For this review, use the dimensioned drawing (mm, ordinates from the lowest corner) and the shaded views. A direction names the side the tool comes from. Coordinates: 2 decimals unless noted, no trailing zeros. Loops run counter-clockwise (first coordinate to the right, second up) from the corner with the lowest first, then second, coordinate; pieces in that order, holes last. Notation, with made-up numbers: M -36,24.5 L -5,24.5 A31 ccw -5,49.5 Z; hole C 84,60 d5. An arc over 180 degrees is marked long. Write each question's results on one line, items separated by ' | '. Start each with the question number.
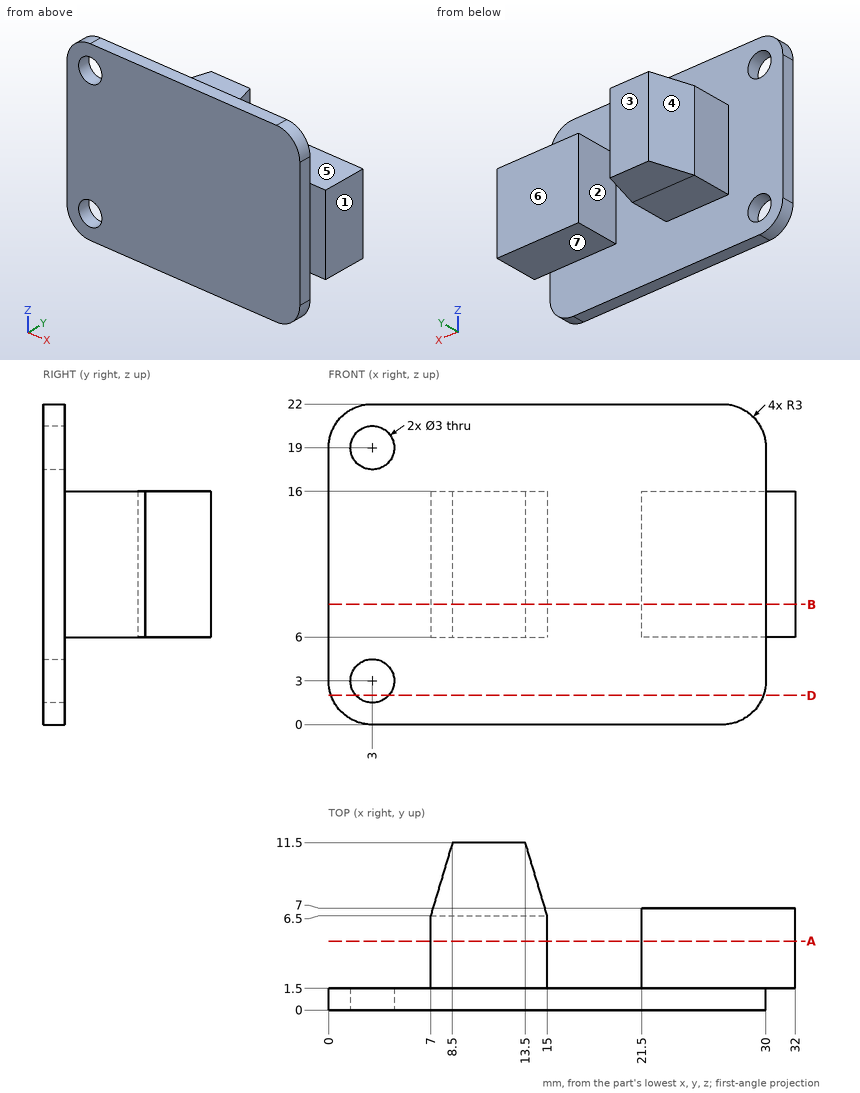
Q1. For the marked faces 5, 6 and 7, list the 3-axis set-ups (+Z, -Z, +X, -X, +Y, -Y) from which the entire face can be reached by the end or side of a thin tool; tool diameter is ignored.
Q2. The part is to be moulded in two halves that separate along X. For the marked faces 1, 2, 3 and 4, say which applies: pulls with the +X half, pulls with the -X half, needs draft (parallel to the pull), parting line crosses it, or undercut.
Q3. Take a section at B-B, the plane z = 8.25. Give the boundary of the cut face in (x, y).
Q4. Insertion check: P1, Ø8, axis at x = 27.5, z = 11, coming from the +Y side; P2, Ø0.6, axis at x = 31, z = 13, coming from the -Y side; P3, Ø2.5, axis at y = 4.5, z = 9.5, coming from the -X side. Each pin has a flat end and moves straight along its axis. Give the tip position at first contact, or say it passes through.
Q5. Take a section at D-D, the plane z = 2. Give the boundary of the cut face in (x, y), then the cut area to 3 significant figures.
Q6. Take a section at A-A, the plane y = 4.75. Give the boundary of the cut face in (x, z).
Q7. To check wall thickness, follow line 1 along X through (y, z) = (3, 11.75); line 2 along X through (y, z) = (0.6, 19); line 3 along Y through (x, z) = (7, 4). State the ranges of each line that lie inside material, in increasing order.
Results:
1) face 5: +Z, +X, -X, +Y | face 6: +Z, -Z, +X, +Y | face 7: -Z, +X, -X, +Y
2) face 1: pulls with the +X half | face 2: undercut | face 3: needs draft | face 4: pulls with the -X half
3) outline: M 0,0 L 30,0 L 30,1.5 L 32,1.5 L 32,7 L 21.5,7 L 21.5,1.5 L 15,1.5 L 15,6.5 L 13.5,11.5 L 8.5,11.5 L 7,6.5 L 7,1.5 L 0,1.5 Z
4) P1: y = 7 | P2: y = 1.5 | P3: x = 7
5) outline: M 0.17,0 L 1.88,0 L 1.88,1.5 L 0.17,1.5 Z; M 4.12,0 L 29.83,0 L 29.83,1.5 L 4.12,1.5 Z | area: 41.1 mm^2
6) outline: M 7,6 L 15,6 L 15,16 L 7,16 Z; M 21.5,6 L 32,6 L 32,16 L 21.5,16 Z
7) line 1: 7 to 15, 21.5 to 32 | line 2: 0 to 1.5, 4.5 to 30 | line 3: 0 to 1.5
